Design review of the part built by this model. Coordinates are the model's own, in mm. Face numbers are marked on the shaded views. A direction names the side the tool comes from. Give positions to 0.01 mm unless a question says otherwise; leave off trailing zeros. Order: outer loops, then holes, each group sorted by start corner. A loop starts at its lowest first (then second) coordinate and runs counter-clockwise, first axis right, second up. Notation, with made-up numbers: (-4, 59.5) -> (28, 59.5) arc R18 cw to (28, 79.5) -> close; hole circle Ø1 at (26, -37.5). An arc over 180 degrees is marked (long way). Return JSON: item names as keys, results as strings.
Solid Edge part; units mm, degrees
sketch "Sketch1" plane through (0, 0, 0) normal (0, 0, 1) x (1, 0, 0)
  line L0 (0, 39.35) -> (39.5, 39.35)
  line L1 (39.5, 0) -> (39.5, 39.35)
  line L2 (0, 0) -> (39.5, 0)
  line L3 (0, 0) -> (0, 39.35)
extrude "Protrusion1" add sketch "Sketch1" along normal blind 19.7
sketch "Sketch2" plane through (0, 19.675, 9.85) normal (-1, 0, 0) x (0, 0, 1)
  line L0 (0, 12.975) -> (-9.85, 12.975)
  line L1 (-9.85, 12.975) -> (-9.85, 9.975)
  line L2 (-9.85, 9.975) -> (9.85, 9.975)
  line L3 (9.85, 9.975) -> (9.85, 12.975)
  line L4 (9.85, 12.975) -> (0, 12.975)
extrude "ExtrudedProtrusion_2" add sketch "Sketch2" along normal blind 7.3
sketch "Sketch3" plane through (39.5, 19.675, 9.85) normal (1, 0, 0) x (0, 0, -1)
  line L0 (-9.85, 12.975) -> (9.85, 12.975)
  line L1 (9.85, 12.975) -> (9.85, 9.975)
  line L2 (9.85, 9.975) -> (-9.85, 9.975)
  line L3 (-9.85, 9.975) -> (-9.85, 12.975)
extrude "ExtrudedProtrusion_3" add sketch "Sketch3" along normal blind 7.3
sketch "Sketch4" plane through (19.75, 39.35, 9.85) normal (0, 1, 0) x (-1, 0, 0)
  line L0 (-7.75, 0) -> (-7.75, 9.85)
  line L1 (-7.75, 9.85) -> (16.25, 9.85)
  line L2 (16.25, 9.85) -> (16.25, -9.85)
  line L3 (16.25, -9.85) -> (-7.75, -9.85)
  line L4 (-7.75, -9.85) -> (-7.75, 0)
extrude "ExtrudedProtrusion_4" add sketch "Sketch4" along normal blind 1
sketch "Sketch5" plane through (15.5, 40.35, 9.85) normal (0, 1, 0) x (-1, 0, 0)
  circle A0 centre (6, 0) radius 2.75
extrude "ExtrudedProtrusion_5" add sketch "Sketch5" along normal blind 5
sketch "Sketch6" plane through (0, 14.825, 9.85) normal (-1, 0, 0) x (0, 0, 1)
  line L0 (-3.75, -13.125) -> (3.75, -13.125)
  line L1 (3.75, -13.125) -> (3.75, -9.525)
  line L2 (3.75, -9.525) -> (-3.75, -9.525)
  line L3 (-3.75, -9.525) -> (-3.75, -13.125)
extrude "ExtrudedProtrusion_6" add sketch "Sketch6" along normal blind 5
sketch "Sketch7" plane through (-3.65, 32.65, 9.85) normal (0, 1, 0) x (0, 0, 1)
  circle A0 centre (-4.75, -1.85) radius 2.1
  circle A1 centre (4.75, -1.85) radius 2.1
extrude "ExtrudedCutout_1" cut sketch "Sketch7" against normal blind 3.8617
sketch "Sketch8" plane through (43.15, 32.65, 9.85) normal (0, 1, 0) x (0, 0, -1)
  circle A0 centre (-4.75, -1.85) radius 2.1
  circle A1 centre (4.75, -1.85) radius 2.1
extrude "Cutout1" cut sketch "Sketch8" against normal up to vertex (3 mm away)
sketch "Sketch9" plane through (19.75, 20.175, 0) normal (0, 0, -1) x (-1, 0, 0)
  line L0 (18.9588, -14.875) -> (-19.75, -14.875)
  line L1 (-19.75, -14.875) -> (-19.75, 9.475)
  line L2 (19.75, 9.4794) -> (-19.75, 9.475)
  line L3 (19.75, -14.875) -> (19.75, 9.4794)
extrude "ExtrudedProtrusion_7" add sketch "Sketch9" along normal blind 0.1 material side at (20.1456, 5.25, 0)
sketch "Sketch10" plane through (0, 14.8272, 9.8) normal (-1, 0, 0) x (0, 0, 1)
  line L0 (-9.8, -9.5272) -> (9.9, -9.5272)
  line L1 (9.9, -9.5272) -> (9.9, 14.8228)
  line L2 (9.9, 14.8228) -> (-9.8, 14.8228)
  line L3 (-9.8, 14.8228) -> (-9.8, -9.5272)
extrude "ExtrudedProtrusion_8" add sketch "Sketch10" along normal blind 0.1
sketch "Sketch11" plane through (19.75, 20.175, 19.7) normal (0, 0, 1) x (1, 0, 0)
  line L0 (-19.75, 9.475) -> (-19.75, -14.875)
  line L1 (-19.75, -14.875) -> (19.75, -14.875)
  line L2 (19.75, -14.875) -> (19.75, 9.475)
  line L3 (19.75, 9.475) -> (-19.75, 9.475)
extrude "ExtrudedProtrusion_9" add sketch "Sketch11" along normal blind 0.1
sketch "Sketch12" plane through (39.5, 14.825, 9.85) normal (1, 0, 0) x (0, 0, -1)
  line L0 (-9.85, 14.825) -> (9.85, 14.825)
  line L1 (9.85, 14.825) -> (9.85, -9.525)
  line L2 (9.85, -9.525) -> (-9.85, -9.525)
  line L3 (-9.85, -9.525) -> (-9.85, 14.825)
extrude "ExtrudedProtrusion_10" add sketch "Sketch12" along normal blind 0.1
properties material "Aluminum Alloy:3.0255 , Al 99.5 , EN-AW 1050A"
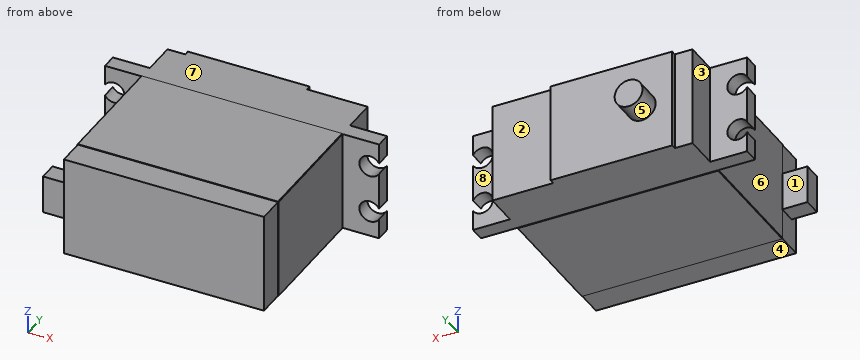
Item 1: Add section B-B (z = 14.6). Give the boundary of the cut face in (x, y).
Result set:
{"outline": "(-3.4, 29.65) -> (-0.1, 29.65) -> (-0.1, 5.3) -> (0, 5.3) -> (0, 0) -> (39.5, 0) -> (39.5, 5.3) -> (39.6, 5.3) -> (39.6, 29.65) -> (42.9, 29.65) -> (42.9, 32.65) -> (39.5, 32.65) -> (39.5, 39.35) -> (27.5, 39.35) -> (27.5, 40.35) -> (3.5, 40.35) -> (3.5, 39.35) -> (0, 39.35) -> (0, 32.65) -> (-3.4, 32.65) -> close"}
Item 2: Add section C-C (y = 37). Give the boundary of the cut face in (x, z), plus the area to 3 significant figures.
Result set:
{"outline": "(0, 0) -> (39.5, 0) -> (39.5, 19.7) -> (0, 19.7) -> close", "area": "778 mm^2"}
Item 3: Wall thickness on L1, parallel to Z at x = 45, y = 30.65; L2, parallel to Y at x = -1, z = 10.5; L3, parallel to Y at x = 19, z = 2: over which ranges is each line inside the solid? List them lowest first. Write a range as [from, to].
Result set:
{"L1": "z = [0, 3], [7.2, 12.5], [16.7, 19.7]", "L2": "y = [1.7, 5.3], [29.65, 32.65]", "L3": "y = [0, 40.35]"}
Item 4: Add section A-A (x = 45). Give the boundary of the cut face in (y, z), plus the area to 3 significant figures.
Result set:
{"outline": "(29.65, 0) -> (32.65, 0) -> (32.65, 3) -> (29.65, 3) -> close; (29.65, 7.2) -> (32.65, 7.2) -> (32.65, 12.5) -> (29.65, 12.5) -> close; (29.65, 16.7) -> (32.65, 16.7) -> (32.65, 19.7) -> (29.65, 19.7) -> close", "area": "33.9 mm^2"}
Item 5: For pin 1 (2 mm diameter, centred on x = 45, z = 8.5, fed in from -Y); pin 2 (0.8 mm diameter, centred on y = 39.5, z = 11, fed in from -X); pin 3 (3.5 mm diameter, centred on y = 34.5, z = 12, fed in from +X), all flat-tipped, find the tip position at first contact; note any pin that passes through.
Result set:
{"pin 1": "stops at y = 29.65", "pin 2": "stops at x = 0", "pin 3": "stops at x = 39.5"}
Item 6: Mouldability with a two-part tool opening along Y and no side actions: class the marked faces 6, 7 and 8 as released by +Y, released by -Y, zero draft, split by the parting line, or undercut.
Result set:
{"face 6": "undercut", "face 7": "zero draft", "face 8": "released by +Y"}
Item 7: Add section D-D (x = 25). Give the boundary of the cut face in (y, z).
Result set:
{"outline": "(0, 0) -> (5.3, 0) -> (5.3, -0.1) -> (29.65, -0.1) -> (29.65, 0) -> (40.35, 0) -> (40.35, 19.7) -> (29.65, 19.7) -> (29.65, 19.8) -> (5.3, 19.8) -> (5.3, 19.7) -> (0, 19.7) -> close"}
Item 8: Machinability: for the marked faces 1, 2, 3, 4 and 5, which of the approach directions +Z, -Z, +X, -X, +Y, -Y give a long, thin tool a straight path to every point of the face, cutting with its end or side? Answer none if there is none.
Result set:
{"face 1": "+Z, -Z, -X", "face 2": "+Z, -Z, +X, +Y", "face 3": "+Z, -Z, -X, +Y", "face 4": "-Z, +X, -X, -Y", "face 5": "+Y"}
